```python
from build123d import *

# Parameters (mm, degrees)
SKETCH1_W                                        = 40.5
SKETCH1_H                                        = 23.5
SKETCH2_R                                        = 5.95
BOSS_EXTRUDE1_DEPTH                              = 10
HOLE1_D                                          = 10.1
HOLE1_DEPTH                                      = 5.2
CBORE_FOR_M4_HEX_HEAD_MACHINE_SCREW1_D           = 4.5
CBORE_FOR_M4_HEX_HEAD_MACHINE_SCREW1_CBORE_D     = 8
CBORE_FOR_M4_HEX_HEAD_MACHINE_SCREW1_CBORE_DEPTH = 6
CHAMFER1_SIZE                                    = 1


with BuildPart() as part:
    # Sketch1 → Revolve1 (revolve)
    with BuildSketch(Plane.XZ, mode=Mode.PRIVATE) as revolve1_sk:
        with Locations((20.25, 11.75)):
            Rectangle(SKETCH1_W, SKETCH1_H)
    revolve(revolve1_sk.sketch.rotate(Axis((0, 0, 23.5), (0, 0, -1)), 180), axis=Axis((0, 0, 23.5), (0, 0, -1)))

    # Sketch2 → Boss-Extrude1 (add)
    with BuildSketch(Plane.XY.offset(23.5)):
        Circle(SKETCH2_R)
    extrude(amount=BOSS_EXTRUDE1_DEPTH)

    # Hole1
    with Locations(Plane.XY.offset(23.5)):
        with Locations((22, 0), (-22, 0)):
            Hole(HOLE1_D / 2, depth=HOLE1_DEPTH)

    # CBORE for M4 Hex Head Machine Screw1 (through all)
    with Locations(Plane.XY.offset(23.5)):
        with Locations((24.748737342, 24.748737342), (-24.748737342, 24.748737342), (24.748737342, -24.748737342), (-24.748737342, -24.748737342)):
            CounterBoreHole(CBORE_FOR_M4_HEX_HEAD_MACHINE_SCREW1_D / 2, CBORE_FOR_M4_HEX_HEAD_MACHINE_SCREW1_CBORE_D / 2, CBORE_FOR_M4_HEX_HEAD_MACHINE_SCREW1_CBORE_DEPTH)

    # Chamfer1
    chamfer1_edges = [part.edges().sort_by_distance(p)[0] for p in [
        (-5.95, 0, 33.5),
    ]]
    chamfer(chamfer1_edges, length=CHAMFER1_SIZE)


solid = part.part
```
CAD build for the part. Positions are in the model's coordinates, mm. A direction names the side the tool comes from. Round coordinates to 2 decimals unless told otherwise and drop trailing zeros. Order: outer loops, then holes, each group sorted by start corner. A loop starts at its lowest first (then second) coordinate and runs counter-clockwise, first axis right, second up. Notation, with made-up numbers: (17.5, -11.5) -> (76.5, -11.5) arc R20 ccw to (76.5, 20.5) -> close; hole circle Ø9 at (-37, 5). An arc over 180 degrees is marked (long way). Write item = value, one per line.
(1) Flat gauge pins, fed straight in: P1, Ø2.5, axis at x = 24.75, y = 24.75, coming from the -Z side; P2, Ø9, axis at x = -23.5, y = -25, coming from the +Z side; P3, Ø4, axis at x = 1.5, z = 28.5, coming from the +Y side; P4, Ø12, axis at y = 6.5, z = 13.5, coming from the -X side. Where does each tip first touch, or does it go through?
Answers follow:
P1 = through
P2 = 23.5
P3 = 5.95
P4 = -40.5
(2) Cut at D-D (y = 10.5). Write the cut outline in (x, z), plus the area to 3 significant figures.
Answers follow:
outline = (-39.12, 0) -> (39.12, 0) -> (39.12, 23.5) -> (-39.12, 23.5) -> close
area = 1,840 mm²
(3) Cut at C-C (z = 19.5). Write the cut outline in (x, y).
Answers follow:
outline = circle Ø81 at (0, 0); hole circle Ø8 at (-24.75, -24.75); hole circle Ø8 at (-24.75, 24.75); hole circle Ø10.1 at (-22, 0); hole circle Ø10.1 at (22, 0); hole circle Ø8 at (24.75, -24.75); hole circle Ø8 at (24.75, 24.75)
(4) Drill centre lines: L1, parallel to Y at x = -24.5, z = 23; L2, parallel to Y at x = 27.5, z = 20.5; L3, parallel to Y at x = 22, z = 20.95. Where is each one in solid material? Low to high.
Answers follow:
L1 = -32.25 to -28.74, -20.76 to -4.39, 4.39 to 20.76, 28.74 to 32.25
L2 = -29.73 to -27.65, -21.85 to 21.85, 27.65 to 29.73
L3 = -34 to -27.65, -21.84 to -5.05, 5.05 to 21.84, 27.65 to 34
(5) 3-axis set-ups, long thin cutter, end or side, ignore diameter. For faces 4 (the cylindrical face through (27.045, 0.222, 20.864)), 5 (the cylindrical face through (-38.63, 12.17, 11.91)): which of +Z, -Z, +X, -X, +Y, -Y reach the whole face in a straight line?
Answers follow:
face_4 = +Z
face_5 = +Z, -Z
(6) Pull direction X, two halves, no side cores. Call faces 1 (the flat face through (-22, 0, 18.3)), 2 (the cylindrical face through (-4.385, 4.021, 27.937)), 3 (the flat face through (-1, -8, 23.5)): +X half, -X half, draft (parallel to the pull), parting line (faces both ways), or undercut.
Answers follow:
face_1 = undercut
face_2 = parting line
face_3 = draft
(7) Cut at A-A (y = 0). Write the cut outline in (x, z), plus the area to 3 significant figures.
Answers follow:
outline = (-40.5, 0) -> (40.5, 0) -> (40.5, 23.5) -> (27.05, 23.5) -> (27.05, 18.3) -> (16.95, 18.3) -> (16.95, 23.5) -> (5.95, 23.5) -> (5.95, 32.5) -> (4.95, 33.5) -> (-4.95, 33.5) -> (-5.95, 32.5) -> (-5.95, 23.5) -> (-16.95, 23.5) -> (-16.95, 18.3) -> (-27.05, 18.3) -> (-27.05, 23.5) -> (-40.5, 23.5) -> close
area = 1,920 mm²
(8) Cut at B-B (x = 0). Write the cut outline in (y, z), plus the area to 3 significant figures.
Answers follow:
outline = (-40.5, 0) -> (40.5, 0) -> (40.5, 23.5) -> (5.95, 23.5) -> (5.95, 32.5) -> (4.95, 33.5) -> (-4.95, 33.5) -> (-5.95, 32.5) -> (-5.95, 23.5) -> (-40.5, 23.5) -> close
area = 2,020 mm²
